Source: CAD feature listing. Evaluate the final solid. Frame: model axes, mm. Coordinates: 2 decimals unless noted, no trailing zeros. Loops run counter-clockwise (first coordinate to the right, second up) from the corner with the lowest first, then second, coordinate; pieces in that order, holes last.
Item 1: Section query C-C, the plane y = 19.75. Return the cut outline in (x, z).
Item 2: Line query: probe 1 along X at (y, z) = (10.75, 0); probe 2 along Z at (x, y) = (0, 20.5); probe 3 along X at (y, z) = (11.75, -4.75). Output: solid intervals per line, ascending.
Item 3: Section query B-B, the plane z = -1.5. Return the cut outline in (x, y), then the cut area to 3 significant figures.
Item 4: Pin query (flat end, axial travel): pin 1 Ø2 at (x, y) = (1.5, 4.5) entering from +Z; pin 2 Ø1 at (y, z) = (14, -7.5) entering from +X; pin 3 Ø2 at (y, z) = (14.5, -2) entering from +X. Return the tip coordinate at first contact, or that it passes through.
Item 5: Section query A-A, the plane x = 0. Return the cut outline in (y, z), then the cut area to 3 significant figures.
Item 6: Section query D-D, the plane z = -7. Return the cut outline in (x, y).
Item 7: Pull-direction query (X, two-part tool) for faces 1 (the flat face through (0, 14, -10.083)), 2 (the cylindrical face through (-0.29, 13.8, -2.23)), 3 (the flat face through (1.25, 14, -7)), 4 (the flat face through (-1.25, 14, -7)); classes: +X half, -X half, draft (parallel to the pull), parting line (faces both ways), or undercut.
```python
from build123d import *

# Parameters (mm, degrees)
SKETCH1_R           = 2.25
BOSS_EXTRUDE1_DEPTH = 28


with BuildPart() as part:
    # Sketch1 → Boss-Extrude1 (new body)
    with BuildSketch(Plane(origin=(0, 0, 0), x_dir=(1, 0, 0), z_dir=(0, 1, 0))):
        with BuildLine():
            Line((1.25, 10.082575695), (-1.25, 10.082575695))
            Line((-1.25, 10.082575695), (-1.25, 4.582575695))
            ThreePointArc((-1.25, 4.582575695), (0, 4.75), (1.25, 4.582575695))
            Line((1.25, 4.582575695), (1.25, 10.082575695))
        make_face()
        with BuildLine():
            Line((1.25, 4.582575695), (-1.25, 4.582575695))
            ThreePointArc((-1.25, 4.582575695), (-2.883140649, -3.774917218), (4.75, 0))
            ThreePointArc((4.75, 0), (3.774917218, 2.883140649), (1.25, 4.582575695))
        make_face()
        Circle(SKETCH1_R, mode=Mode.SUBTRACT)
        with BuildLine():
            ThreePointArc((1.25, 4.582575695), (0, 4.75), (-1.25, 4.582575695))
            Line((-1.25, 4.582575695), (1.25, 4.582575695))
        make_face()
    extrude(amount=BOSS_EXTRUDE1_DEPTH)


solid = part.part
```
Verdict:
1. outline: (-1.25, -10.08) - (1.25, -10.08) - (1.25, -4.58) arc R4.75 ccw (long way) to (-1.25, -4.58) - close; hole circle Ø4.5 at (0, 0)
2. probe 1: x = -4.75 to -2.25, 2.25 to 4.75
2. probe 2: z = -10.08 to -2.25, 2.25 to 4.75
2. probe 3: x = -1.25 to 1.25
3. outline: (-4.51, 0) - (-1.68, 0) - (-1.68, 28) - (-4.51, 28) - close; (1.68, 0) - (4.51, 0) - (4.51, 28) - (1.68, 28) - close
3. area: 158 mm2
4. pin 1: stops at z = 4.72
4. pin 2: stops at x = 1.25
4. pin 3: stops at x = 4.64
5. outline: (0, -10.08) - (28, -10.08) - (28, -2.25) - (0, -2.25) - close; (0, 2.25) - (28, 2.25) - (28, 4.75) - (0, 4.75) - close
5. area: 289 mm2
6. outline: (-1.25, 0) - (1.25, 0) - (1.25, 28) - (-1.25, 28) - close
7. face 1: draft
7. face 2: undercut
7. face 3: +X half
7. face 4: -X half
